Model file for the job. Use its own axes, mm. Face numbers are marked on the shaded views. A direction names the side the tool comes from. Coordinates: 2 decimals unless noted, no trailing zeros. Loops run counter-clockwise (first coordinate to the right, second up) from the corner with the lowest first, then second, coordinate; pieces in that order, holes last.
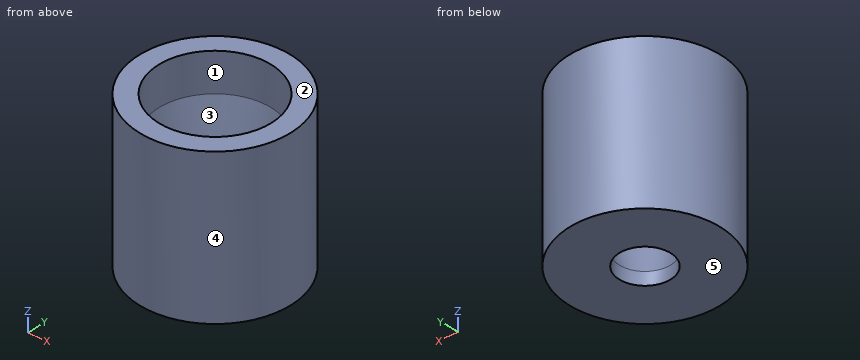
from build123d import *

# Parameters (mm, degrees)
F0_R        = 5.9
F0_R_2      = 2
F1_DEPTH    = 9
F2_SIZE2    = 2.4
F2_SIZE     = 8
F1_FACE_R   = 5.9
F1_FACE_R_2 = 4.4
F3_DEPTH    = 3


with BuildPart() as f1:
    # F0 (on Top) → F1 (new body)
    with BuildSketch(Plane.XY):
        Circle(F0_R)
        Circle(F0_R_2, mode=Mode.SUBTRACT)
    extrude(amount=F1_DEPTH)

    # F2
    f2_edges = [f1.edges().sort_by_distance(p)[0] for p in [
        (-2, 0, 9),
    ]]
    chamfer(f2_edges, length=F2_SIZE, length2=F2_SIZE2)

    # F1_face (on face) → F3 (join)
    with BuildSketch(Plane.XY.offset(9)):
        Circle(F1_FACE_R)
        Circle(F1_FACE_R_2, mode=Mode.SUBTRACT)
    extrude(amount=F3_DEPTH)


solid = f1.part
Q1. Slice it at A-A (y = 0). List the corners of the cut face in (x, z).
Answers:
outline: (-5.9, 0) - (-2, 0) - (-2, 1) - (-4.4, 9) - (-4.4, 12) - (-5.9, 12) - close; (2, 0) - (5.9, 0) - (5.9, 12) - (4.4, 12) - (4.4, 9) - (2, 1) - close
Q2. Mould opens along Y. For the marked faces 3, 4 and 5 say: +Y half, -Y half, draft (parallel to the pull), parting line (faces both ways), or undercut.
Answers:
face 3: undercut
face 4: parting line
face 5: draft
Q3. Flat gauge pins, fed straight in: P1, Ø2, axis at y = 4, z = 8, coming from the -X side; P2, Ø1, axis at x = -2.5, z = 9, coming from the +Y side. Where does each tip first touch, or does it go through?
Answers:
P1: stops at x = -5.08
P2: stops at y = 5.55
Q4. Slice it at C-C (z = 6.5). List the corners of the cut face in (x, y), and give its area (3 significant figures).
Answers:
outline: circle Ø11.8 at (0, 0); hole circle Ø7.3 at (0, 0)
area: 67.5 mm2
Q5. Slice it at D-D (z = 4). List the corners of the cut face in (x, y).
Answers:
outline: circle Ø11.8 at (0, 0); hole circle Ø5.8 at (0, 0)
Q6. Which spindle directions (+Z, -Z, +X, -X, +Y, -Y) get a long thin tool onto all of the face, cutting with end or side? Do the marked faces 1 and 2. Say none if no direction does.
Answers:
face 1: +Z
face 2: +Z, +X, -X, +Y, -Y
Q7. Drill centre lines: line 1 (Y direction, x = 0, z = 10.5); line 2 (Y direction, x = 0, z = 0.7); line 3 (X direction, y = 1.75, z = 10.5). Where is each one in solid material? Low to high.
Answers:
line 1: y = -5.9 to -4.4, 4.4 to 5.9
line 2: y = -5.9 to -2, 2 to 5.9
line 3: x = -5.63 to -4.04, 4.04 to 5.63
